The listing builds one solid part. Answer for the finished solid, in the listing's coordinates (mm). A direction names the side the tool comes from. Coordinates: 2 decimals unless noted, no trailing zeros. Write each loop counter-clockwise with the first axis right and the second up, starting at its lowest first coordinate (ties: lowest second). Pieces come first, ordered by that corner, then holes. Notation, with made-up numbers: M 63,10.25 L 112,10.25 A8 ccw 112,25.25 Z; hole C 1,7.25 d7. An arc over 180 degrees is marked long. Write item = value, one per line. Start each with the question number.
Autodesk Fusion 360 part; units mm, degrees
sketch "Sketch5" plane through (0, 0, 0) normal (0, 0, 1) x (1, 0, 0)
  circle A0 centre (0, 0) radius 12.5
  circle A1 centre (0, 0) radius 10
  circle A2 centre (0, 0) radius 7.5
  dimension "d32" = 25
  dimension "d33" = 20
  dimension "d34" = 15
extrude "Extrude8" add sketch "Sketch5" along normal blind 10 contours A0
extrude "Extrude9" add sketch "Sketch5" along normal blind 16 contours A1
sketch "Sketch6" plane through (0, 0, 0) normal (1, 0, 0) x (0, 0, -1)
  line L0 (0, 0) -> (100, 0)
  line L1 (100, 0) -> (100, 7)
  line L2 (0, 12.5) -> (0, -12.5)
  line L3 (100, 7) -> (21.3505, 7)
  line L4 (0, 12.5) -> (10.3963, 8.8615)
  arc A0 (10.3963, 8.8615) -> (21.3505, 7) centre (21.3505, 40.1609) ccw
  dimension "d39" = 100
  dimension "d40" = 7
  dimension "d43" = 33.1609
revolve "Revolve2" add sketch "Sketch6" angle 360 about axis through (0, 0, 0) along (0, 0, -1)
sketch "Sketch7" plane through (0, 0, -100) normal (0, 0, -1) x (-1, 0, 0)
  circle A0 centre (0, 0) radius 7
  line L0 (-1.5, 2) -> (1.5, 2)
  arc A1 (-1.5, 2) -> (1.5, 2) centre (0, 0) ccw
  dimension "d1" = 5
extrude "Extrude10" cut sketch "Sketch7" against normal blind 15 contours L0 A1
extrude "Extrude11" add 1 faces at (-1.613, 0.9883, 0) along direction (0, 0, 1) blind 11
1. Each of these flat-tipped pins is pushed along its axis until it touches: pin 1 (3 mm diameter, centred on x = 0, y = 0, fed in from +Z); pin 2 (8 mm diameter, centred on y = -8.5, z = -58, fed in from -X); pin 3 (4 mm diameter, centred on x = 4.5, z = -64, fed in from -Y); pin 4 (13.5 mm diameter, centred on x = 0, y = 0, fed in from -Z). Where does it stop, or does it pass through?
2. For a pull along Y with two mould halves and no side action, classify faces 4 (the face through (-7.493, -0.33, 13.465)), 5 (the face through (-3, 0, -100)), 6 (the face through (-2.17, 9.76, 12.96)) as pulls with the +Y half, pulls with the -Y half, needs draft (parallel to the pull), parting line crosses it, or undercut.
3. The part is cut by section C-C, the plane x = 0. Write down the section's boundary in (y, z), and give its area (3 significant figures).
4. The part is cut by section A-A, the plane z = -92. Write down the section's boundary in (x, y), and give its area (3 significant figures).
5. Straight lines are drawn through the part: L1, parallel to Y at x = 0, z = 13.55; L2, parallel to X at y = 0, z = -94.5; L3, parallel to Z at x = 2, y = -5.75. For each, find the intervals that lie inside material, in ascending order. Write a range as [from, to].
6. The part is cut by section D-D, the plane z = -47. Write down the section's boundary in (x, y).
7. For faces 1 (the face through (11.923, -3.755, 4.93)), 2 (the face through (2.681, 6.466, -60.125)), 3 (the face through (0, 0, 11)), determine the directions among +Z, -Z, +X, -X, +Y, -Y from which every point of the face is accessible in a straight line to the end or side of a thin tool.
8. The part is cut by section B-B, the plane y = 0. Write down the section's boundary in (x, z).
Solution:
q1.pin_1 = 11
q1.pin_2 = -5.36
q1.pin_3 = -6.54
q1.pin_4 = -100
q2.face_4 = undercut
q2.face_5 = needs draft
q2.face_6 = parting line crosses it
q3.outline = M -12.5,0 L -8.86,-10.4 A33.16 cw -7,-21.35 L -7,-100 L -2.5,-100 L -2.5,-85 L 2,-85 L 2,-100 L 7,-100 L 7,-21.35 A33.16 cw 8.86,-10.4 L 12.5,0 L 12.5,10 L 10,10 L 10,16 L 7.5,16 L 7.5,11 L -7.5,11 L -7.5,16 L -10,16 L -10,10 L -12.5,10 Z
q3.area = 1,720 mm^2
q4.outline = C 0,0 d14; hole M -1.5,2 A2.5 ccw long 1.5,2 Z
q4.area = 135 mm^2
q5.L1 = [-10, -7.5], [7.5, 10]
q5.L2 = [-7, -2.5], [2.5, 7]
q5.L3 = [-100, 11]
q6.outline = C 0,0 d14
q7.face_1 = +Z, -Z
q7.face_2 = -Z
q7.face_3 = +Z
q8.outline = M -12.5,0 L -8.86,-10.4 A33.16 cw -7,-21.35 L -7,-100 L -2.5,-100 L -2.5,-85 L 2.5,-85 L 2.5,-100 L 7,-100 L 7,-21.35 A33.16 cw 8.86,-10.4 L 12.5,0 L 12.5,10 L 10,10 L 10,16 L 7.5,16 L 7.5,11 L -7.5,11 L -7.5,16 L -10,16 L -10,10 L -12.5,10 Z
